Verification items for this drawing (mm, ordinates from the low corner). Round coordinates to 2 decimals unless told otherwise and drop trailing zeros. Order: outer loops, then holes, each group sorted by start corner. A loop starts at its lowest first (then second) coordinate and runs counter-clockwise, first axis right, second up. Notation, with made-up numbers: (22.5, 32) - (72.5, 32) arc R11 cw to (72.5, 40) - close; hole circle Ø6 at (-38.5, 6). An arc over 180 degrees is marked (long way). Return JSON: item names as keys, results as strings. Group by question number.
Q1. Sectioned sample at D-D, the plane x = 16. Record the cut outline in (y, z).
Q2. Sectioned sample at C-C, the plane y = 21. Record the cut outline in (x, z).
Q3. Sectioned sample at B-B, the plane z = 20. Record the cut outline in (x, y).
Q4. Draft check along X on the marked faces 1, 2, 3 and 4. Enter one of: pulls with the +X half, pulls with the -X half, needs draft (parallel to the pull), parting line crosses it, or undercut.
Q5. Gauge pin test, flat ends, axial feed: pin 1 Ø4.5 at (x, z) = (12.56, 6.56) entering from -Y; pin 2 Ø2.5 at (x, y) = (5.5, 31.5) entering from -Z; pin 3 Ø6 at (x, y) = (46, 8) entering from +Z. Record the tip position at first contact, or that the pin passes through.
Q6. Material ranges on line 1 along Y through (x, z) = (46, 9.25); line 2 along X through (y, z) = (2, 18.5); line 3 along X through (y, z) = (30, 4), recorded low to high.
Q7. Sectioned sample at A-A, the plane x = 26. Record the cut outline in (y, z), then the cut area to 3 significant figures.
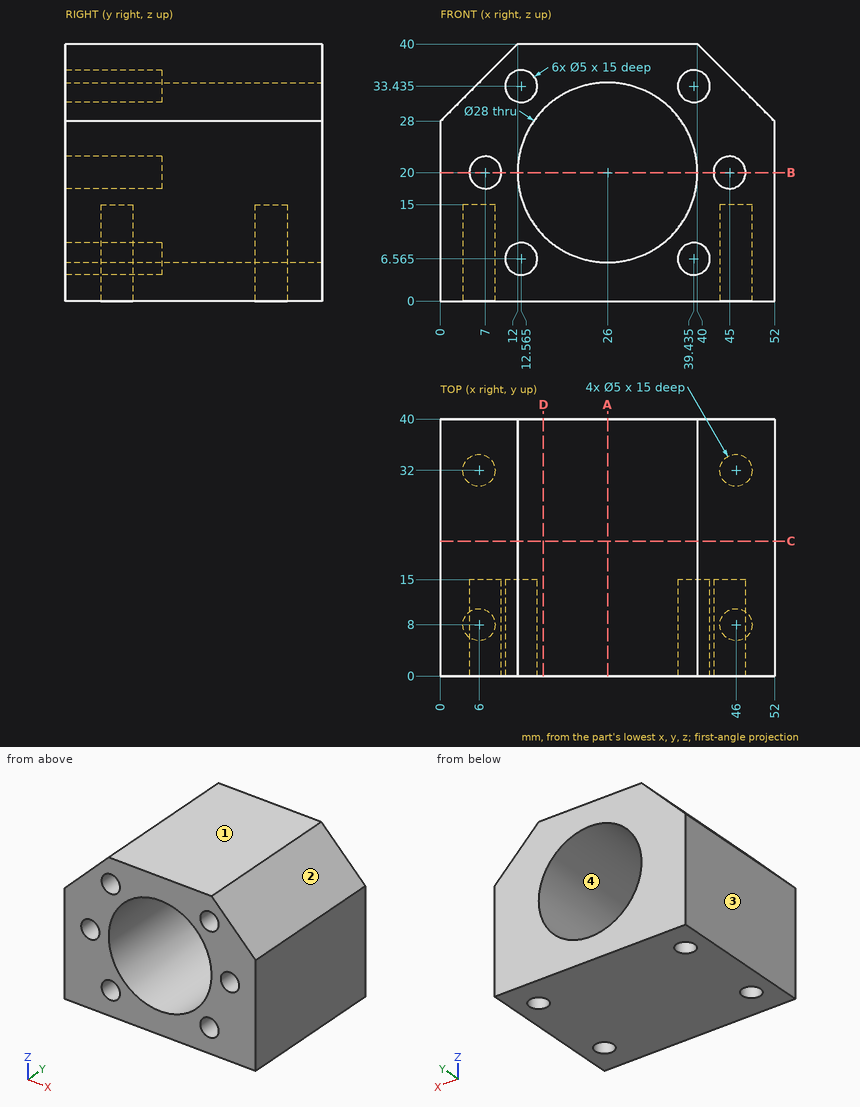
Reply:
{
 "1": {"outline": "(0, 0) - (40, 0) - (40, 10.2) - (0, 10.2) - close; (0, 29.8) - (40, 29.8) - (40, 40) - (0, 40) - close"},
 "2": {"outline": "(0, 0) - (52, 0) - (52, 28) - (40, 40) - (12, 40) - (0, 28) - close; hole circle Ø28 at (26, 20)"},
 "3": {"outline": "(0, 0) - (4.5, 0) - (4.5, 15) - (9.5, 15) - (9.5, 0) - (12, 0) - (12, 40) - (0, 40) - close; (40, 0) - (42.5, 0) - (42.5, 15) - (47.5, 15) - (47.5, 0) - (52, 0) - (52, 40) - (40, 40) - close"},
 "4": {"face 1": "needs draft", "face 2": "pulls with the +X half", "face 3": "pulls with the -X half", "face 4": "undercut"},
 "5": {"pin 1": "y = 15", "pin 2": "z = 15", "pin 3": "z = 37"},
 "6": {"line 1": "0 to 5.5, 10.5 to 29.5, 34.5 to 40", "line 2": "0 to 5, 9 to 12.08, 39.92 to 43, 47 to 52", "line 3": "0 to 4.5, 7.5 to 44.5, 47.5 to 52"},
 "7": {"outline": "(0, 0) - (40, 0) - (40, 6) - (0, 6) - close; (0, 34) - (40, 34) - (40, 40) - (0, 40) - close", "area": "480 mm^2"}
}
